For this review, take the finished solid that the model builds, in its own axes (mm). A direction names the side the tool comes from. Coordinates: 2 decimals unless noted, no trailing zeros. Order: outer loops, then holes, each group sorted by start corner. A loop starts at its lowest first (then second) coordinate and runs counter-clockwise, first axis right, second up. Notation, with made-up numbers: (65.25, 2) -> (88.25, 2) arc R25 ccw to (88.25, 22) -> close; hole circle Ø7 at (20.25, -7). An arc over 180 degrees is marked (long way). Return JSON: item names as keys, results as strings. Group by question number.
Item 1: For line 1 along X through (y, z) = (62, 2.35); line 2 along Y through (x, z) = (5, 2.75); line 3 along Y through (x, z) = (62, 7.1), list the stretches that pass through material, from the lowest coordinate up.
Item 2: Draft analysis for pull direction Y (two halves, no side actions). For faces 1 (the flat face through (12, 62, 7)), 2 (the flat face through (62, -2, 5)), 3 (the flat face through (62, -10, 8)), 4 (the cylindrical face through (64.385, -4.249, 7.535)), state which applies: +Y half, -Y half, draft (parallel to the pull), parting line (faces both ways), or undercut.
Item 3: Take a section at A-A (x = 5). Write out the cut boundary in (y, z), then the cut area to 3 significant figures.
Item 4: Machinability: for faces 5 (the flat face through (42, -5, 8)), 6 (the flat face through (6, 83, 7)), 7 (the flat face through (82, -5, 8)), 8 (the flat face through (115, 62, 4)), which of the approach directions +Z, -Z, +X, -X, +Y, -Y give a long, thin tool a straight path to every point of the face, cutting with its end or side? Answer none if there is none.
Item 5: Take a section at B-B (y = -5). Write out the cut boundary in (x, z).
Item 6: Take a section at D-D (y = 53.5). Write out the cut boundary in (x, z).
Item 7: Insertion check: pin 1 (2 mm diameter, centred on x = 19, z = 4.5, fed in from -Y); pin 2 (1 mm diameter, centred on y = 87.5, z = 2.5, fed in from -X); pin 3 (2.5 mm diameter, centred on y = -5, z = 6.5, fed in from -X); pin 4 (2.5 mm diameter, centred on y = -3.5, z = 6.5, fed in from +X). Each pin has a flat end and moves straight along its axis. Give the tip position at first contact, or say it passes through.
Item 8: Take a section at C-C (z = 8). Write out the cut boundary in (x, y), then the cut area to 3 significant figures.
Autodesk Inventor part; units mm, degrees
ref_plane "YZ Plane" through (0, 0, 0) normal (1, 0, 0) x (0, 1, 0)
ref_plane "XZ Plane" through (0, 0, 0) normal (0, 1, 0) x (-1, 0, 0)
ref_plane "XY Plane" through (0, 0, 0) normal (0, 0, 1) x (1, 0, 0)
sketch "Sketch1" plane through (0, 0, 0) normal (0, 0, 1) x (1, 0, 0)
  line L0 (0, 0) -> (124, 0)
  line L1 (124, 0) -> (124, 124)
  line L2 (124, 124) -> (0, 124)
  line L3 (0, 124) -> (0, 0)
  circle A0 centre (5, 62) radius 2.5
  circle A1 centre (119, 62) radius 2.5
  point P0 (124, 62)
  point P1 (0, 62)
  dimension "d0" = 124
  dimension "d1" = 124
  dimension "d2" = 5
  dimension "d3" = 5
  dimension "d4" = 5
  dimension "d5" = 5
extrude "Extrusion1" add sketch "Sketch1" along normal blind 10
sketch "Sketch2" plane through (0, 0, 10) normal (0, 0, 1) x (1, 0, 0)
  line L0 (42, 0) -> (82, 0)
  line L1 (82, 0) -> (82, -10)
  line L2 (82, -10) -> (42, -10)
  line L3 (42, -10) -> (42, 0)
  circle A0 centre (62, -5) radius 2.5
  line L4 (0, 0) -> (124, 0)
  point P0 (82, -5)
  point P1 (62, -10)
  point P2 (62, 0)
  dimension "d8" = 40
  dimension "d9" = 10
  dimension "d10" = 5
extrude "Extrusion2" add sketch "Sketch2" against normal blind 5
sketch "Sketch3" plane through (0, 0, 10) normal (0, 0, 1) x (1, 0, 0)
  line L0 (0, 124) -> (0, 0)
  line L1 (0, 83) -> (12, 83)
  line L2 (12, 83) -> (12, 41)
  line L3 (12, 41) -> (0, 41)
  line L4 (0, 41) -> (0, 83)
  line L5 (124, 0) -> (124, 124)
  line L6 (124, 41) -> (112, 41)
  line L7 (112, 41) -> (112, 83)
  line L8 (112, 83) -> (124, 83)
  line L9 (124, 83) -> (124, 41)
  point P0 (124, 62)
  point P1 (124, 62)
  dimension "d13" = 12
  dimension "d14" = 42
  dimension "d15" = 12
  dimension "d16" = 42
extrude "Extrusion3" cut sketch "Sketch3" against normal blind 6
sketch "Sketch4" plane through (0, 0, 10) normal (0, 0, 1) x (1, 0, 0)
  line L0 (0, 124) -> (0, 0)
  line L1 (0, 124) -> (124, 124)
  line L2 (124, 124) -> (124, 130)
  line L3 (124, 130) -> (0, 130)
  line L4 (0, 130) -> (0, 124)
  dimension "d19" = 6
extrude "Extrusion4" add sketch "Sketch4" against normal blind 10
properties part number "TC008" material "ABS Plastic"
Findings below:
{
 "1": {"line 1": "x = 0 to 2.5, 7.5 to 116.5, 121.5 to 124", "line 2": "y = 0 to 59.5, 64.5 to 130", "line 3": "y = -10 to -7.5, -2.5 to 130"},
 "2": {"face 1": "undercut", "face 2": "draft", "face 3": "-Y half", "face 4": "undercut"},
 "3": {"outline": "(0, 0) -> (59.5, 0) -> (59.5, 4) -> (41, 4) -> (41, 10) -> (0, 10) -> close; (64.5, 0) -> (130, 0) -> (130, 10) -> (83, 10) -> (83, 4) -> (64.5, 4) -> close", "area": "1,030 mm2"},
 "4": {"face 5": "+Z, -Z, -X, -Y", "face 6": "+Z, -X", "face 7": "+Z, -Z, +X, -Y", "face 8": "+Z, +X"},
 "5": {"outline": "(42, 5) -> (59.5, 5) -> (59.5, 10) -> (42, 10) -> close; (64.5, 5) -> (82, 5) -> (82, 10) -> (64.5, 10) -> close"},
 "6": {"outline": "(0, 0) -> (124, 0) -> (124, 4) -> (112, 4) -> (112, 10) -> (12, 10) -> (12, 4) -> (0, 4) -> close"},
 "7": {"pin 1": "stops at y = 0", "pin 2": "stops at x = 0", "pin 3": "stops at x = 42", "pin 4": "stops at x = 82"},
 "8": {"outline": "(0, 0) -> (42, 0) -> (42, -10) -> (82, -10) -> (82, 0) -> (124, 0) -> (124, 41) -> (112, 41) -> (112, 83) -> (124, 83) -> (124, 130) -> (0, 130) -> (0, 83) -> (12, 83) -> (12, 41) -> (0, 41) -> close; hole circle Ø5 at (62, -5)", "area": "15,500 mm2"}
}
